Could you check a few things on this model? Use its own coordinates, in mm. A direction names the side the tool comes from. Give positions to 0.01 mm unless a question says otherwise; leave off trailing zeros. Loops run counter-clockwise (first coordinate to the right, second up) from the corner with the lowest first, then second, coordinate; pieces in that order, holes last. Notation, with made-up numbers: M 24.5,-5.5 L 41.5,-5.5 A30 cw 41.5,17.5 Z; hole C 74,-10.5 d5. An arc over 180 degrees is marked long. Use CSV: the item, a comma, the result in double quotes.
```python
from build123d import *

# Parameters (mm, degrees)
SKETCH1_W           = 44
SKETCH1_H           = 64
SKETCH1_W_2         = 40
SKETCH1_H_2         = 60
SKETCH1_W_3         = 37
SKETCH1_H_3         = 57
BOSS_EXTRUDE1_DEPTH = 2.5
SKETCH2_W           = 44
SKETCH2_H           = 64
SKETCH2_W_2         = 41
SKETCH2_H_2         = 61
BOSS_EXTRUDE2_DEPTH = 14
SKETCH3_W           = 44
SKETCH3_H           = 64
BOSS_EXTRUDE3_DEPTH = 1
SKETCH4_W           = 8
SKETCH4_H           = 5
CUT_EXTRUDE1_DEPTH  = 8
SKETCH5_R           = 2.5
CUT_EXTRUDE2_DEPTH  = 8
FILLET1_R           = 2


with BuildPart() as part:
    # Sketch1 → Boss-Extrude1 (new body)
    # profile 1 of 2: a face of its own
    with BuildSketch(Plane(origin=(0, 0, 0), x_dir=(1, 0, 0), z_dir=(0, 1, 0))):
        Rectangle(SKETCH1_W, SKETCH1_H)
        Rectangle(SKETCH1_W_2, SKETCH1_H_2, mode=Mode.SUBTRACT)
    # profile 2 of 2: a face of its own
    with BuildSketch(Plane(origin=(0, 0, 0), x_dir=(1, 0, 0), z_dir=(0, 1, 0))):
        Rectangle(SKETCH1_W_2, SKETCH1_H_2)
        Rectangle(SKETCH1_W_3, SKETCH1_H_3, mode=Mode.SUBTRACT)
    extrude(amount=-BOSS_EXTRUDE1_DEPTH)

    # Sketch2 → Boss-Extrude2 (add)
    with BuildSketch(Plane(origin=(0, 0, 0), x_dir=(1, 0, 0), z_dir=(0, 1, 0))):
        Rectangle(SKETCH2_W, SKETCH2_H)
        Rectangle(SKETCH2_W_2, SKETCH2_H_2, mode=Mode.SUBTRACT)
    extrude(amount=BOSS_EXTRUDE2_DEPTH)

    # Sketch3 → Boss-Extrude3 (add)
    with BuildSketch(Plane.XZ.offset(2.5)):
        Rectangle(SKETCH3_W, SKETCH3_H)
    extrude(amount=BOSS_EXTRUDE3_DEPTH)

    # Sketch4 → Cut-Extrude1 (cut)
    with BuildSketch(Plane(origin=(-20.5, 0, 0), x_dir=(0, 0, -1), z_dir=(1, 0, 0))):
        with Locations((0.298083895, 4)):
            Rectangle(SKETCH4_W, SKETCH4_H)
    extrude(amount=-CUT_EXTRUDE1_DEPTH, mode=Mode.SUBTRACT)

    # Sketch5 → Cut-Extrude2 (cut)
    with BuildSketch(Plane(origin=(0, 0, 30.5), x_dir=(-1, 0, 0), z_dir=(0, 0, -1))):
        with Locations((15.5, 4)):
            Circle(SKETCH5_R)
    extrude(amount=-CUT_EXTRUDE2_DEPTH, mode=Mode.SUBTRACT)

    # Fillet1
    fillet1_edges = [part.edges().sort_by_distance(p)[0] for p in [
        (-22, 5.25, -32),
        (22, 5.25, -32),
        (22, 5.25, 32),
        (-22, 5.25, 32),
    ]]
    fillet(fillet1_edges, radius=FILLET1_R)


solid = part.part
```
1. If we mould it in two halves opening along Z, with no side actions, what happens to faces 1 (the face through (-21.43, 5.37, 31.4)), 2 (the face through (0, 7, -30.5)), 3 (the face through (21.4, 5.13, -31.43)), 4 (the face through (0, -3.5, 0))? For each: +Z half, -Z half, draft (parallel to the pull), parting line (faces both ways), or undercut.
Outcome:
face 1,"+Z half"
face 2,"undercut"
face 3,"-Z half"
face 4,"draft"
2. Please list where these lines run through material, in increasing order: line 1 (Z direction, x = -3, y = 6.5); line 2 (X direction, y = -1.75, z = -1.5); line 3 (Z direction, x = 14.5, y = -1.75).
Outcome:
line 1,"-32 to -30.5, 30.5 to 32"
line 2,"-22 to -18.5, 18.5 to 22"
line 3,"-32 to -28.5, 28.5 to 32"
3. I'm going to push flat-ended pins straight in: pin 1 Ø1.6 at (x, y) = (-21, 3.5) entering from -Z; pin 2 Ø18.5 at (x, z) = (-1.5, -10) entering from +Y; pin 3 Ø3 at (x, z) = (-17.5, -23.5) entering from +Y. Where does each tip first touch, or does it pass through?
Outcome:
pin 1,"z = -31.99"
pin 2,"y = -2.5"
pin 3,"y = 0"
4. I want a section at D-D, the plane z = -16.5. List the corners of the cut face in (x, y) for me, then the cut area to 4 significant figures.
Outcome:
outline,"M -22,-3.5 L 22,-3.5 L 22,14 L 20.5,14 L 20.5,0 L 18.5,0 L 18.5,-2.5 L -18.5,-2.5 L -18.5,0 L -20.5,0 L -20.5,14 L -22,14 Z"
area,"103.5 mm2"
5. I want a section at B-B, the plane x = -15.5. List the corners of the cut face in (y, z) for me, then the cut area to 3 significant figures.
Outcome:
outline,"M -3.5,-32 L 14,-32 L 14,-30.5 L 0,-30.5 L 0,-28.5 L -2.5,-28.5 L -2.5,28.5 L 0,28.5 L 0,30.5 L 1.5,30.5 L 1.5,32 L -3.5,32 Z; M 6.5,30.5 L 14,30.5 L 14,32 L 6.5,32 Z"
area,"116 mm2"
6. I want a section at C-C, the plane y = 4. List the corners of the cut face in (x, z) for me.
Outcome:
outline,"M -22,-30 A2 ccw -20,-32 L 20,-32 A2 ccw 22,-30 L 22,30 A2 ccw 20,32 L -13,32 L -13,30.5 L 20.5,30.5 L 20.5,-30.5 L -20.5,-30.5 L -20.5,-4.3 L -22,-4.3 Z; M -22,3.7 L -20.5,3.7 L -20.5,30.5 L -18,30.5 L -18,32 L -20,32 A2 ccw -22,30 Z"
7. Which directions (+Z, -Z, +X, -X, +Y, -Y) give clear straight access to the entire face, cutting with the end or side of a thin tool? Please do faces 5 (the face through (-21, 1.5, 0)), 6 (the face through (18.5, -1, 0)), 7 (the face through (-13, 4, 31)).
Outcome:
face 5,"-X"
face 6,"+Y"
face 7,"+Z"
8. I want a section at A-A, the plane y = 8. List the corners of the cut face in (x, z) for me, then the cut area to 3 significant figures.
Outcome:
outline,"M -22,-30 A2 ccw -20,-32 L 20,-32 A2 ccw 22,-30 L 22,30 A2 ccw 20,32 L -20,32 A2 ccw -22,30 Z; hole M -20.5,-30.5 L 20.5,-30.5 L 20.5,30.5 L -20.5,30.5 Z"
area,"312 mm2"
